```python
from build123d import *

# Parameters (mm, degrees)
F0_R     = 1.375
F0_R_2   = 6.95
F1_DEPTH = 1.5


with BuildPart() as f1:
    # F0 (on Top) → F1 (new body, symmetric)
    with BuildSketch(Plane.XY):
        with BuildLine():
            Line((-31, -19.5), (-27.8, -19.5))
            add(Edge.make_bspline(
                [(-27.8, -19.5), (-18.5333333333, -18.25), (0, -15.75), (18.5333333333, -18.25), (27.8, -19.5)],
                knots=[0, 0, 0, 0, 0.5, 1, 1, 1, 1], degree=3))
            Line((27.8, -19.5), (31, -19.5))
            add(Edge.make_bspline(
                [(39.8, 0), (37.8467765607, -1.8901869566), (33.4188629122, -6.1751983155), (31.8671997538, -14.7228525715), (31, -19.5)],
                knots=[0, 0, 0, 0, 0.4411159734, 1, 1, 1, 1], degree=3))
            add(Edge.make_bspline(
                [(31, 19.5), (31.8282806058, 14.7207922386), (33.3126793566, 6.1557600729), (37.8114855459, 1.8868834383), (39.8, 0)],
                knots=[0, 0, 0, 0, 0.5579906379, 1, 1, 1, 1], degree=3))
            Line((31, 19.5), (27.8, 19.5))
            Line((27.8, 19.5), (-27.8, 19.5))
            Line((-27.8, 19.5), (-31, 19.5))
            add(Edge.make_bspline(
                [(-31, 19.5), (-31.8282806058, 14.7207922386), (-33.3126793566, 6.1557600729), (-37.8114855459, 1.8868834383), (-39.8, 0)],
                knots=[0, 0, 0, 0, 0.5579906379, 1, 1, 1, 1], degree=3))
            add(Edge.make_bspline(
                [(-31, -19.5), (-31.8671997538, -14.7228525715), (-33.4188629122, -6.1751983155), (-37.8467765607, -1.8901869566), (-39.8, 0)],
                knots=[0, 0, 0, 0, 0.5588840266, 1, 1, 1, 1], degree=3))
        make_face()
        with Locations((-20.85, -14.625)):
            Circle(F0_R, mode=Mode.SUBTRACT)
        with Locations((-13.9, -14.625)):
            Circle(F0_R, mode=Mode.SUBTRACT)
        with Locations((-6.95, -14.625)):
            Circle(F0_R, mode=Mode.SUBTRACT)
        with Locations((-20.85, -9.75)):
            Circle(F0_R, mode=Mode.SUBTRACT)
        Polygon((-27.8, -3.3), (-27.8, -6.5), (-31, -6.5), (-31, -3.3), (-31, -1.5), (-27.8, -1.5), align=None, mode=Mode.SUBTRACT)
        with Locations((-20.85, -4.875)):
            Circle(F0_R, mode=Mode.SUBTRACT)
        with Locations((-13.9, -9.75)):
            Circle(F0_R, mode=Mode.SUBTRACT)
        with Locations((-6.95, -9.75)):
            Circle(F0_R, mode=Mode.SUBTRACT)
        with Locations((-13.9, -4.875)):
            Circle(F0_R, mode=Mode.SUBTRACT)
        with Locations((0, -14.625)):
            Circle(F0_R, mode=Mode.SUBTRACT)
        with Locations((6.95, -14.625)):
            Circle(F0_R, mode=Mode.SUBTRACT)
        with Locations((13.9, -14.625)):
            Circle(F0_R, mode=Mode.SUBTRACT)
        with Locations((20.85, -14.625)):
            Circle(F0_R, mode=Mode.SUBTRACT)
        with Locations((0, -9.75)):
            Circle(F0_R, mode=Mode.SUBTRACT)
        with Locations((6.95, -9.75)):
            Circle(F0_R, mode=Mode.SUBTRACT)
        with Locations((13.9, -9.75)):
            Circle(F0_R, mode=Mode.SUBTRACT)
        with Locations((13.9, -4.875)):
            Circle(F0_R, mode=Mode.SUBTRACT)
        with Locations((20.85, -9.75)):
            Circle(F0_R, mode=Mode.SUBTRACT)
        with Locations((20.85, -4.875)):
            Circle(F0_R, mode=Mode.SUBTRACT)
        Polygon((31, -3.3), (31, -6.5), (27.8, -6.5), (27.8, -4.875), (27.8, -3.3), (27.8, -1.5), (31, -1.5), align=None, mode=Mode.SUBTRACT)
        with Locations((-20.85, 0)):
            Circle(F0_R, mode=Mode.SUBTRACT)
        Polygon((-27.8, 1.8441202119), (-27.8, 1.5), (-31, 1.5), (-31, 3.6441202119), (-31, 6.5), (-27.8, 6.5), (-27.8, 4.875), align=None, mode=Mode.SUBTRACT)
        with Locations((-20.85, 4.875)):
            Circle(F0_R, mode=Mode.SUBTRACT)
        with Locations((-13.9, 0)):
            Circle(F0_R, mode=Mode.SUBTRACT)
        with Locations((-13.9, 4.875)):
            Circle(F0_R, mode=Mode.SUBTRACT)
        with Locations((-20.85, 9.75)):
            Circle(F0_R, mode=Mode.SUBTRACT)
        with Locations((-20.85, 14.625)):
            Circle(F0_R, mode=Mode.SUBTRACT)
        with Locations((-13.9, 9.75)):
            Circle(F0_R, mode=Mode.SUBTRACT)
        with Locations((-6.95, 9.75)):
            Circle(F0_R, mode=Mode.SUBTRACT)
        with Locations((-13.9, 14.625)):
            Circle(F0_R, mode=Mode.SUBTRACT)
        with Locations((-6.95, 14.625)):
            Circle(F0_R, mode=Mode.SUBTRACT)
        Circle(F0_R_2, mode=Mode.SUBTRACT)
        with Locations((13.9, 0)):
            Circle(F0_R, mode=Mode.SUBTRACT)
        with Locations((13.9, 4.875)):
            Circle(F0_R, mode=Mode.SUBTRACT)
        with Locations((20.85, 0)):
            Circle(F0_R, mode=Mode.SUBTRACT)
        Polygon((27.8, 3.3), (27.8, 6.5), (31, 6.5), (31, 1.5), (27.8, 1.5), align=None, mode=Mode.SUBTRACT)
        with Locations((20.85, 4.875)):
            Circle(F0_R, mode=Mode.SUBTRACT)
        with Locations((0, 9.75)):
            Circle(F0_R, mode=Mode.SUBTRACT)
        with Locations((6.95, 9.75)):
            Circle(F0_R, mode=Mode.SUBTRACT)
        with Locations((13.9, 9.75)):
            Circle(F0_R, mode=Mode.SUBTRACT)
        with Locations((0, 14.625)):
            Circle(F0_R, mode=Mode.SUBTRACT)
        with Locations((6.95, 14.625)):
            Circle(F0_R, mode=Mode.SUBTRACT)
        with Locations((13.9, 14.625)):
            Circle(F0_R, mode=Mode.SUBTRACT)
        with Locations((20.85, 9.75)):
            Circle(F0_R, mode=Mode.SUBTRACT)
        with Locations((20.85, 14.625)):
            Circle(F0_R, mode=Mode.SUBTRACT)
    extrude(amount=F1_DEPTH, both=True)


solid = f1.part
```
Read the model definition and answer for the solid it produces. Units are mm, in the model's axes. Coordinates: 2 decimals unless noted, no trailing zeros. Write each loop counter-clockwise with the first axis right and the second up, starting at its lowest first coordinate (ties: lowest second). Pieces come first, ordered by that corner, then holes. Notation, with made-up numbers: (83.5, 8) - (140.5, 8) arc R29 ccw to (140.5, 43) - close; hole circle Ø11 at (-11.5, -38). An arc over 180 degrees is marked (long way). Answer as a JSON object with one key per item and string values. Group by question number.
1. Each of these flat-tipped pins is pushed along its axis until it touches: P1, Ø1.6, axis at x = 20.85, y = 4.875, coming from the +Z side; P2, Ø1, axis at y = -9.5, z = 0, coming from the -X side; P3, Ø1, axis at x = -12, z = 0, coming from the -Y side. Where does it stop, or does it pass through?
2. A cutting plane is placed at A-A (x = 30). Determine the outline of the cut face in (y, z).
3. Consider L1, parallel to X at y = -2, z = 1.2; L2, parallel to X at y = 2.5, z = -0.4; L3, parallel to Y at x = -8, z = -0.2. Determine where each line is inside the solid, lowest interval first. Write a range as [from, to].
4. A cutting plane is placed at B-B (x = 0). Give the number of separate pieces and of enclosed holes in the cut face, plus the area to 3 significant figures.
Worked out:
{
 "1": {"P1": "passes through", "P2": "stops at x = -33.44", "P3": "stops at y = -17.64"},
 "2": {"outline": "(-19.5, -1.5) - (-6.5, -1.5) - (-6.5, 1.5) - (-19.5, 1.5) - close; (-1.5, -1.5) - (1.5, -1.5) - (1.5, 1.5) - (-1.5, 1.5) - close; (6.5, -1.5) - (19.5, -1.5) - (19.5, 1.5) - (6.5, 1.5) - close"},
 "3": {"L1": "x = [-37.79, -31], [-27.8, -6.66], [6.66, 27.8], [31, 37.79]", "L2": "x = [-37.28, -31], [-27.8, -6.48], [6.48, 27.8], [31, 37.28]", "L3": "y = [-17.28, -15.51], [-13.74, -10.64], [-8.86, 8.86], [10.64, 13.74], [15.51, 19.5]"},
 "4": {"separate pieces": "6", "enclosed holes": "0", "area": "34.8 mm²"}
}
